from build123d import *

# Parameters (mm, degrees)
F0_W     = 76.2
F0_H     = 114.652204
F2_DEPTH = 127
F3_R     = 12.7
F1_T     = -2.54


with BuildPart() as f2:
    # F0 (on Front) → F2 (new body)
    with BuildSketch(Plane.XZ):
        with BuildLine():
            Line((-38.1, -57.326102), (-38.1, 57.326102))
            ThreePointArc((-38.1, 57.326102), (-95.426102, 0), (-38.1, -57.326102))
        make_face()
        Rectangle(F0_W, F0_H)
    extrude(amount=F2_DEPTH)

    # F3
    f3_edges = [f2.edges().sort_by_distance(p)[0] for p in [
        (-95.426102, -127, 0),
    ]]
    fillet(f3_edges, radius=F3_R)

    # F1
    f1_openings = [f2.faces().sort_by_distance(p)[0] for p in [
        (38.1, -63.210212, 0),
        (-23.187149, 0, 0),
    ]]
    offset(amount=F1_T, openings=f1_openings)


solid = f2.part
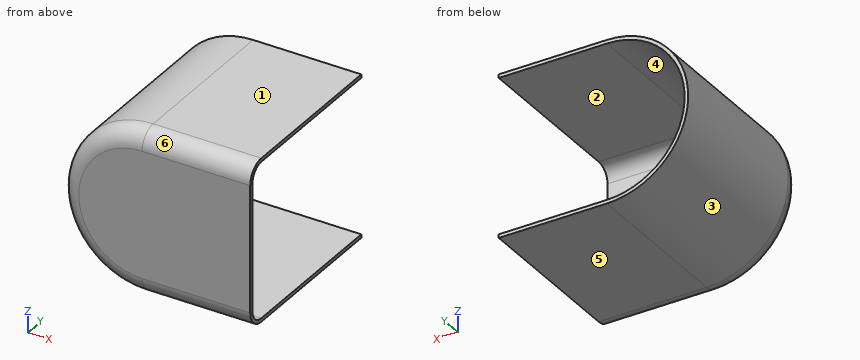
Could you check a few things on this model? Use its own coordinates, in mm. Face numbers are marked on the shaded views. A direction names the side the tool comes from. Round coordinates to 2 decimals unless told otherwise and drop trailing zeros. Order: outer loops, then holes, each group sorted by start corner. A loop starts at its lowest first (then second) coordinate and runs counter-clockwise, first axis right, second up.
(1) Imagine slicing it at B-B (z = 0). Write out the boundary of the cut face in (x, y), plus the area to 3 significant figures.
Response values:
outline: (-95.43, -114.3) arc R12.7 ccw to (-82.73, -127) - (38.1, -127) - (38.1, -124.46) - (-82.73, -124.46) arc R10.16 cw to (-92.89, -114.3) - (-92.89, 0) - (-95.43, 0) - close
area: 643 mm2
(2) Which directions (+Z, -Z, +X, -X, +Y, -Y) give clear straight access to the entire face, cutting with the end or side of a thin tool? Please do the marked faces 1 and 2.
Response values:
face 1: +Z, +X, -X, +Y, -Y
face 2: +X, +Y
(3) If we mould it in two halves opening along Z, with no side actions, what happens to the marked faces 3, 4, 5 and 6? For each: released by +Z, released by -Z, zero draft, split by the parting line, or undercut.
Response values:
face 3: split by the parting line
face 4: undercut
face 5: released by -Z
face 6: released by +Z
(4) I'm going to push flat-ended pins straight in: pin 1 (3 mm diameter, centred on x = -76, y = -68, fed in from +Z); pin 2 (1 mm diameter, centred on y = -75, z = 12.5, fed in from +X); pin 3 (1.5 mm diameter, centred on y = -37, z = 30, fed in from +X). Where does each tip first touch, or does it pass through?
Response values:
pin 1: stops at z = 44.29
pin 2: stops at x = -91.32
pin 3: stops at x = -83.44
(5) Please list where these lines run through material, in increasing order: line 1 along Z through (x, y) = (-19, -20.5); line 2 along Y through (x, z) = (31.5, 3); line 3 along Z through (x, y) = (13, -120.5).
Response values:
line 1: z = -57.33 to -54.79, 54.79 to 57.33
line 2: y = -127 to -124.46
line 3: z = -55.71 to -52.68, 52.68 to 55.71
(6) Imagine slicing it at A-A (y = -19.5). Write out the boundary of the cut face in (x, z), plus the area to 3 significant figures.
Response values:
outline: (-38.1, -57.33) - (38.1, -57.33) - (38.1, -54.79) - (-38.1, -54.79) arc R54.79 cw to (-38.1, 54.79) - (38.1, 54.79) - (38.1, 57.33) - (-38.1, 57.33) arc R57.33 ccw to start
area: 834 mm2
(7) Imagine slicing it at C-C (x = 16.5). Write out the boundary of the cut face in (y, z).
Response values:
outline: (-127, -44.63) arc R12.7 ccw to (-114.3, -57.33) - (0, -57.33) - (0, -54.79) - (-114.3, -54.79) arc R10.16 cw to (-124.46, -44.63) - (-124.46, 44.63) arc R10.16 cw to (-114.3, 54.79) - (0, 54.79) - (0, 57.33) - (-114.3, 57.33) arc R12.7 ccw to (-127, 44.63) - close
